from build123d import *

# Parameters (mm, degrees)
SKIZZE1_W                       = 28.05
SKIZZE1_H                       = 30.0045
AUFSATZ_LINEAR_AUSTRAGEN1_DEPTH = 20.05
VERRUNDUNG1_R                   = 6
SKIZZE2_R                       = 1.65
AUFSATZ_LINEAR_AUSTRAGEN2_DEPTH = 15.5
VERRUNDUNG1_OF_SPIEGELN1_R      = 6


with BuildPart() as part:
    # Skizze1 → Aufsatz-Linear austragen1 (new body)
    with BuildSketch(Plane(origin=(0, 0, 0), x_dir=(0, 0, -1), z_dir=(1, 0, 0))):
        with Locations((-14.025, 0)):
            Rectangle(SKIZZE1_W, SKIZZE1_H)
    aufsatz_linear_austragen1 = extrude(amount=AUFSATZ_LINEAR_AUSTRAGEN1_DEPTH)

    # Verrundung1
    verrundung1_edges = [part.edges().sort_by_distance(p)[0] for p in [
        (10.025, -15.00225, 28.05),
        (10.025, 15.00225, 28.05),
    ]]
    fillet(verrundung1_edges, radius=VERRUNDUNG1_R)

    # Skizze2 → Aufsatz-Linear austragen2 (add)
    with BuildSketch(Plane(origin=(20.05, 0, 0), x_dir=(0, 0, -1), z_dir=(1, 0, 0))):
        with Locations(Location((-14.025, 10, 0), (0, 0, 180))):
            Circle(SKIZZE2_R)
        with Locations(Location((-14.025, -10, 0), (0, 0, 180))):
            Circle(SKIZZE2_R)
    aufsatz_linear_austragen2 = extrude(amount=AUFSATZ_LINEAR_AUSTRAGEN2_DEPTH)

    # Skizze3 → Rotation1 (revolve)
    with BuildSketch(Plane.XY.offset(14.025), mode=Mode.PRIVATE) as rotation1_sk:
        Polygon((35.55, 10), (36.541420021, 10), (35.55, 11.65), align=None)
    rotation1 = revolve(rotation1_sk.sketch.rotate(Axis((35.55, 10, 14.025), (-1, 0, 0)), 270), axis=Axis((35.55, 10, 14.025), (-1, 0, 0)))

    # Skizze4 → Rotation2 (revolve)
    with BuildSketch(Plane.XY.offset(14.025), mode=Mode.PRIVATE) as rotation2_sk:
        Polygon((35.55, -10), (36.541420021, -10), (35.55, -8.35), align=None)
    rotation2 = revolve(rotation2_sk.sketch.rotate(Axis((35.55, -10, 14.025), (-1, 0, 0)), 270), axis=Axis((35.55, -10, 14.025), (-1, 0, 0)))

    # Spiegeln1: Aufsatz-Linear austragen1, Aufsatz-Linear austragen2, Rotation1, Rotation2 across plane
    add(aufsatz_linear_austragen1.mirror(Plane.ZY))
    add(aufsatz_linear_austragen2.mirror(Plane.ZY))
    add(rotation1.mirror(Plane.ZY))
    add(rotation2.mirror(Plane.ZY))

    # Verrundung1 of Spiegeln1
    verrundung1_of_spiegeln1_edges = [part.edges().sort_by_distance(p)[0] for p in [
        (-10.025, -15.00225, 28.05),
        (-10.025, 15.00225, 28.05),
    ]]
    fillet(verrundung1_of_spiegeln1_edges, radius=VERRUNDUNG1_OF_SPIEGELN1_R)


solid = part.part
Input: part model. Units: mm. Frame: model coordinates. A direction names the side the tool comes from. Coordinates: 2 decimals unless noted, no trailing zeros. Order: outer loops, then holes, each group sorted by start corner. A loop starts at its lowest first (then second) coordinate and runs counter-clockwise, first axis right, second up.
1. Access query for faces 1 (the cylindrical face through (-27.69, 11.61, 13.67)), 2 (the flat face through (0, 15.002, 11)), 3 (the cylindrical face through (27.69, 11.61, 13.67)). Directions: +Z, -Z, +X, -X, +Y, -Y. A direction counts if a zero-diameter tool reaches every point of the face in a straight line with its end or side. Return the directions, or none.
Checked values:
face 1: -X
face 2: +Z, -Z, +X, -X, +Y
face 3: +X
2. Cut plane A-A, the plane x = -31. Return loops of the section in (y, z) (3 decimals).
Checked values:
outline: circle Ø3.3 at (-10, 14.025); circle Ø3.3 at (10, 14.025)
3. Ray query, line 1 along X through (y, z) = (5, 25); line 2 along Y through (x, z) = (-11.5, 25.5); line 3 along Z through (x, y) = (-22.5, -9.5). Return the intervals inside material, ascending.
Checked values:
line 1: x = -20.05 to 20.05
line 2: y = -13.91 to 13.91
line 3: z = 12.45 to 15.6
4. Draft query along Y for faces 4 (the cylindrical face through (-10.165, 13.198, 26.339)), 5 (the conical face through (36.37, 10.28, 13.99)), 6 (the cylindrical face through (-10.165, -13.198, 26.339)). Return one class per face: +Y half, -Y half, draft (parallel to the pull), parting line (faces both ways), or undercut.
Checked values:
face 4: +Y half
face 5: undercut
face 6: -Y half
5. Contact query for flat-ended pins moving along their axis: P1, Ø1, axis at x = 28.5, y = 10, coming from the +Z side (3 decimals); P2, Ø6, axis at x = 23.5, y = 6.5, coming from the -Z side; P3, Ø5, axis at y = -2, z = 15, coming from the -X side. Output: stop coordinate, or through.
Checked values:
P1: stops at z = 15.675
P2: stops at z = 12.45
P3: stops at x = -20.05
6. Cut plane D-D, the plane y = 3.5. Return loops of the section in (x, z).
Checked values:
outline: (-20.05, 0) - (20.05, 0) - (20.05, 28.05) - (-20.05, 28.05) - close
7. Cut plane B-B, the plane z = 5. Return loops of the section in (x, y), plus the area to 3 significant figures.
Checked values:
outline: (-20.05, -15) - (20.05, -15) - (20.05, 15) - (-20.05, 15) - close
area: 1,200 mm2
8. Cut plane C-C, the plane x = -19. Return loops of the section in (y, z).
Checked values:
outline: (-15, 0) - (15, 0) - (15, 22.05) arc R6 ccw to (9, 28.05) - (-9, 28.05) arc R6 ccw to (-15, 22.05) - close
